```python
from build123d import *

# Parameters (mm, degrees)
SKETCH2_W          = 34
SKETCH2_H          = 34
CUT_EXTRUDE1_DEPTH = 11


with BuildPart() as part:
    # Sketch1 → Revolve1 (revolve)
    with BuildSketch(Plane.XY):
        Polygon((0, 0), (63, 0), (69, 10), (65.501428863, 10), (61.301428863, 3), (0, 3), align=None)
    revolve(axis=Axis((0, 0, 0), (0, 1, 0)))

    # Sketch2 → Cut-Extrude1 (cut, through all)
    with BuildSketch(Plane.XZ):
        with Locations((6, 29)):
            Rectangle(SKETCH2_W, SKETCH2_H)
    extrude(amount=-CUT_EXTRUDE1_DEPTH, mode=Mode.SUBTRACT)


solid = part.part
```
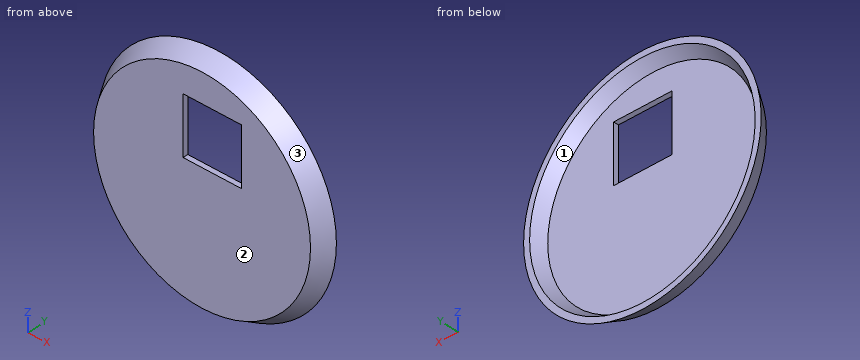
For this review, take the finished solid that the model builds, in its own axes (mm). Face numbers are marked on the shaded views. Round coordinates to 2 decimals unless told otherwise and drop trailing zeros. Write each loop counter-clockwise with the first axis right and the second up, starting at its lowest first coordinate (ties: lowest second). Pieces come first, ordered by that corner, then holes. Notation, with made-up numbers: (67, 41) - (94, 41) arc R8 cw to (94, 45) - close; hole circle Ø8 at (60, 66). An arc over 180 degrees is marked (long way). Answer as a JSON object with one key per item and string values.
1. We need section C-C on y = 5. Give the boundary of the cut face in (x, z).
Response values:
{"outline": "circle Ø132 at (0, 0); hole circle Ø125 at (0, 0)"}
2. We need section B-B on z = 0. Give the boundary of the cut face in (x, y).
Response values:
{"outline": "(-69, 10) - (-63, 0) - (63, 0) - (69, 10) - (65.5, 10) - (61.3, 3) - (-61.3, 3) - (-65.5, 10) - close"}
3. To check wall thickness, follow line 1 along Z through (x, y) = (-53, 8.5); line 2 along Y through (x, z) = (-2.5, -30.5); line 3 along Z through (x, y) = (45.5, 8). State the ranges of each line that lie inside material, in increasing order.
Response values:
{"line 1": "z = -42.76 to -36.94, 36.94 to 42.76", "line 2": "y = 0 to 3", "line 3": "z = -50.27 to -45.44, 45.44 to 50.27"}
4. Draft analysis for pull direction Z (two halves, no side actions). For the marked faces 1, 2 and 3, state which applies: +Z half, -Z half, draft (parallel to the pull), parting line (faces both ways), or undercut.
Response values:
{"face 1": "undercut", "face 2": "draft", "face 3": "parting line"}
5. We need section A-A on x = 0. Give the boundary of the cut face in (y, z).
Response values:
{"outline": "(0, -63) - (10, -69) - (10, -65.5) - (3, -61.3) - (3, 12) - (0, 12) - close; (0, 46) - (3, 46) - (3, 61.3) - (10, 65.5) - (10, 69) - (0, 63) - close"}
6. For pin 1 Ø1.5 at (x, y) = (28, 4) entering from -Z; pin 2 Ø1.5 at (x, z) = (-41.5, -39) entering from -Y; pin 3 Ø3 at (y, z) = (5, 28) entering from -X; pin 4 Ø5 at (x, y) = (5.5, 7.5) entering from +Z, all flat-tipped, find the tip position at first contact; note any pin that passes through.
Response values:
{"pin 1": "stops at z = -59.71", "pin 2": "stops at y = 0", "pin 3": "stops at x = -60.97", "pin 4": "stops at z = 68.79"}
